CAD build for the part. Positions are in the model's coordinates, mm. A direction names the side the tool comes from. Round coordinates to 2 decimals unless told otherwise and drop trailing zeros. Loops run counter-clockwise (first coordinate to the right, second up) from the corner with the lowest first, then second, coordinate; pieces in that order, holes last. Notation, with made-up numbers: M -17.75,-1.75 L -5.75,-1.75 A30 cw -5.75,33.25 Z; hole C 22.25,-22.5 d9. An arc over 180 degrees is marked long. Use a Markdown table: item, result. Add a question column.
(1) Wall check: L1, parallel to Y at x = 13, z = 4; L2, parallel to Y at x = -11, z = 0.75; L3, parallel to X at y = 131, z = -1. Give the ranges that are in metal, low to high.
(2) Flat gauge pins, fed straight in: P1, Ø10, axis at x = -13.5, y = 68, coming from the -Z side; P2, Ø1.5, axis at x = 16, z = -1, coming from the -Y side; P3, Ø1.5, axis at x = -14.5, z = -2.5, coming from the +Y side; P4, Ø4, axis at y = 155, z = -3, coming from the +X side. Where does each tip first touch, or does it go through?
(3) Band-saw the part on A-A, the plane x = 16.5. Write the cut outline in (y, z).
(4) Two-plate mould, pull along Z, no slides. Class faces 1 (the face through (13, 0, 0)), 2 (the face through (9.304, 11.711, -0.07)), 3 (the face through (0, 156, -5)), 4 (the face through (-13, 0, 0)): released by +Z, released by -Z, zero draft, split by the parting line, or undercut.
(5) Which spindle directions (+Z, -Z, +X, -X, +Y, -Y) get a long thin tool onto all of the face, cutting with end or side? Do faces 5 (the face through (-16, 10, 0)), 6 (the face through (7.5, 109, 0)), 7 (the face through (0, 156, 5)). Say none if no direction does.
(6) Band-saw the part on B-B, the plane y = 189. Write the cut outline in (x, z), and give its area (3 significant figures).
from build123d import *

# Parameters (mm, degrees)
PAD_DEPTH       = 5
SKETCH001_R     = 6.35
POCKET_DEPTH    = 50.001
POCKET001_DEPTH = 10.001
CHAMFER_SIZE    = 2
FILLET_R        = 6


with BuildPart() as part:
    # Sketch → Pad (new body, symmetric)
    with BuildSketch(Plane.XY):
        with BuildLine():
            ThreePointArc((7.5, 204.15152), (0, 253), (-7.5, 204.15152))
            Line((-7.5, 204.15152), (-7.5, 10))
            Line((-25, 10), (-7.5, 10))
            Line((-25, -5), (-25, 10))
            Line((25, -5), (-25, -5))
            Line((25, 10), (25, -5))
            Line((7.5, 10), (25, 10))
            Line((7.5, 204.15152), (7.5, 10))
        make_face()
    extrude(amount=PAD_DEPTH, both=True)

    # Sketch001 → Pocket (cut, through all)
    with BuildSketch(Plane(origin=(-25, 0, 0), x_dir=(0, -1, 0), z_dir=(-1, 0, 0))):
        with Locations((6.35, 0)):
            Circle(SKETCH001_R)
    extrude(amount=-POCKET_DEPTH, mode=Mode.SUBTRACT)

    # Sketch002 → Pocket001 (cut, through all)
    with BuildSketch(Plane.XY.offset(5)):
        Polygon((0, 2), (-10, -15.320508), (10, -15.320508), align=None)
    extrude(amount=-POCKET001_DEPTH, mode=Mode.SUBTRACT)

    # Chamfer
    chamfer_edges = [part.edges().sort_by_distance(p)[0] for p in [
        (13.780448, -2.435603, 5),
        (-13.780448, -2.435603, 5),
        (-25, 0, 0),
        (-1.154701, 0, 0),
        (1.154701, 0, 0),
        (25, 0, 0),
        (13.780448, -2.435603, -5),
        (-13.780448, -2.435603, -5),
    ]]
    chamfer(chamfer_edges, length=CHAMFER_SIZE)

    # Fillet
    fillet_edges = [part.edges().sort_by_distance(p)[0] for p in [
        (25, 10, 0),
        (7.5, 10, 0),
        (-7.5, 10, 0),
        (-25, 10, 0),
        (7.5, 204.15152, 0),
        (-7.5, 204.15152, 0),
    ]]
    fillet(fillet_edges, radius=FILLET_R)


solid = part.part
Return value:
| question | item | result |
|---|---|---|
| 1 | L1 | -0.87 to 10.02, 206.65 to 249.35 |
| 1 | L2 | -0.04 to 10.55, 205.55 to 250.45 |
| 1 | L3 | -7.5 to 7.5 |
| 2 | P1 | through |
| 2 | P2 | y = -0.25 |
| 2 | P3 | y = 248.88 |
| 2 | P4 | x = 7.5 |
| 3 | outline | M -1.07,-3.53 L -0.44,-5 L 10,-5 L 10,5 L -0.44,5 L -1.07,3.53 A6.35 cw Z; M 209.22,-5 L 246.78,-5 L 246.78,5 L 209.22,5 Z |
| 4 | face 1 | undercut |
| 4 | face 2 | zero draft |
| 4 | face 3 | released by -Z |
| 4 | face 4 | undercut |
| 5 | face 5 | +Z, -Z, -X |
| 5 | face 6 | +Z, -Z, +X |
| 5 | face 7 | +Z, +X, -X, +Y, -Y |
| 6 | outline | M -7.5,-5 L 7.5,-5 L 7.5,5 L -7.5,5 Z |
| 6 | area | 150 mm^2 |
